from build123d import *
from OCP.BRepFilletAPI import BRepFilletAPI_MakeChamfer

# Parameters (mm, degrees)
SKETCH_1_W          = 24
SKETCH_1_H          = 107
EXTRUDE_1_DEPTH     = 15
EXTRUDE_2_DEPTH     = 9
SKETCH_3_W          = 20
SKETCH_3_H          = 20
EXTRUDE_4_DEPTH     = 40
SKETCH_4_W          = 24
SKETCH_4_H          = 12
EXTRUDE_6_DEPTH     = 25
CHAMFER_2_SIZE      = 2
SKETCH_5_W          = 16
SKETCH_5_H          = 16
SKETCH_5_R          = 3
EXTRUDE_7_DEPTH     = 10
CHAMFER_3_SIZE      = 2
SKETCH_6_W          = 24
SKETCH_6_H          = 12
SKETCH_6_R          = 2.1
EXTRUDE_8_DEPTH     = 12
EXTRUDE_START       = -12
SKETCH_7_W          = 24
SKETCH_7_H          = 12
SKETCH_7_R          = 2.1
EXTRUDE_9_DEPTH     = 12
FILLET_1_R          = 10
CHAMFER_4_SIZE      = 16
CHAMFER_4_SIZE2     = 27.712812921
CUT_EXTRUDE_1_DEPTH = 12
FILLET_2_R          = 2


with BuildPart() as part:
    # Эскиз1 → Бобышка-Вытянуть1 (new body)
    with BuildSketch(Plane(origin=(0, 0, 0), x_dir=(1, 0, 0), z_dir=(0, 1, 0))):
        with Locations((-12, 0)):
            Rectangle(SKETCH_1_W, SKETCH_1_H)
    extrude(amount=EXTRUDE_1_DEPTH)

    # Эскиз2 → Бобышка-Вытянуть2 (add)
    with BuildSketch(Plane(origin=(0, 15, 0), x_dir=(1, 0, 0), z_dir=(0, 1, 0))):
        Polygon((0, 0), (0, 41.5), (-24, 41.5), (-24, -41.5), (0, -41.5), align=None)
    extrude(amount=EXTRUDE_2_DEPTH)

    # Эскиз3 → Бобышка-Вытянуть4 (add)
    with BuildSketch(Plane(origin=(0, 0, 0), x_dir=(1, 0, 0), z_dir=(0, 1, 0))):
        Polygon((0, 53.5), (20, 41.5), (0, 41.5), align=None)
        with Locations((10, 31.5)):
            Rectangle(SKETCH_3_W, SKETCH_3_H)
        with Locations((10, -31.5)):
            Rectangle(SKETCH_3_W, SKETCH_3_H)
        Polygon((0, -41.5), (0, -53.5), (20, -41.5), align=None)
    extrude(amount=EXTRUDE_4_DEPTH)

    # Эскиз4 → Бобышка-Вытянуть6 (add)
    with BuildSketch(Plane(origin=(0, 15, 0), x_dir=(1, 0, 0), z_dir=(0, 1, 0))):
        with Locations((-12, 47.5)):
            Rectangle(SKETCH_4_W, SKETCH_4_H)
        with Locations((-12, -47.5)):
            Rectangle(SKETCH_4_W, SKETCH_4_H)
    extrude(amount=EXTRUDE_6_DEPTH)

    # Фаска2
    chamfer_2_edges = [part.edges().sort_by_distance(p)[0] for p in [
        (0, 12, -21.5),
        (20, 20, -21.5),
        (0, 12, 21.5),
        (20, 20, 21.5),
    ]]
    chamfer(chamfer_2_edges, length=CHAMFER_2_SIZE)

    # Эскиз5 → Бобышка-Вытянуть7 (add)
    # profile 1 of 3: a face of its own
    with BuildSketch(Plane(origin=(0, 0, 0), x_dir=(1, 0, 0), z_dir=(0, 1, 0))):
        with Locations((-32, 45.5)):
            Rectangle(SKETCH_5_W, SKETCH_5_H)
        with Locations(Location((-32, 45.5, 0), (0, 0, 270))):
            Circle(SKETCH_5_R, mode=Mode.SUBTRACT)
    # profile 2 of 3: a face of its own
    with BuildSketch(Plane(origin=(0, 0, 0), x_dir=(1, 0, 0), z_dir=(0, 1, 0))):
        with Locations((-32, -45.5)):
            Rectangle(SKETCH_5_W, SKETCH_5_H)
        with Locations(Location((-32, -45.5, 0), (0, 0, 270))):
            Circle(SKETCH_5_R, mode=Mode.SUBTRACT)
    # profile 3 of 3: a face of its own
    with BuildSketch(Plane(origin=(0, 0, 0), x_dir=(1, 0, 0), z_dir=(0, 1, 0))):
        with Locations((8, 0)):
            Rectangle(SKETCH_5_W, SKETCH_5_H)
        with Locations(Location((8, 0, 0), (0, 0, 270))):
            Circle(SKETCH_5_R, mode=Mode.SUBTRACT)
    extrude(amount=EXTRUDE_7_DEPTH)

    # Фаска3
    chamfer_3_edges = [part.edges().sort_by_distance(p)[0] for p in [
        (-24, 10, -45.5),
        (-24, 10, 45.5),
        (0, 10, 0),
    ]]
    chamfer(chamfer_3_edges, length=CHAMFER_3_SIZE)

    # Эскиз6 → Бобышка-Вытянуть8 (add)
    with BuildSketch(Plane(origin=(0, 0, -53.5), x_dir=(-1, 0, 0), z_dir=(0, 0, -1))):
        with Locations((12, 46)):
            Rectangle(SKETCH_6_W, SKETCH_6_H)
        with Locations((12, 46)):
            Circle(SKETCH_6_R, mode=Mode.SUBTRACT)
    extrude(amount=-EXTRUDE_8_DEPTH)

    # Эскиз7 → Бобышка-Вытянуть9 (add)
    with BuildSketch(Plane.XY.offset(53.5).offset(EXTRUDE_START)):
        with Locations((-12, 46)):
            Rectangle(SKETCH_7_W, SKETCH_7_H)
        with Locations(Location((-12, 46, 0), (0, 0, 180))):
            Circle(SKETCH_7_R, mode=Mode.SUBTRACT)
    extrude(amount=EXTRUDE_9_DEPTH)

    # Скругление1
    fillet_1_edges = [part.edges().sort_by_distance(p)[0] for p in [
        (0, 52, -47.5),
        (-24, 52, -47.5),
        (-24, 52, 47.5),
        (0, 52, 47.5),
    ]]
    fillet(fillet_1_edges, radius=FILLET_1_R)

    # Фаска4: one chamfer whose edges measure the first distance from different faces: ONE call of the kernel's chamfer builder (chamfer() names one face for all edges)
    chamfer_4_edges_1 = [part.edges().sort_by_distance(p)[0] for p in [
        (20, 40, 32.5),
    ]]
    chamfer_4_side_1 = [part.faces().sort_by_distance(p)[0] for p in [
        (9.191763192, 40, 34.779279279),
    ]]
    chamfer_4_edges_2 = [part.edges().sort_by_distance(p)[0] for p in [
        (20, 40, -32.5),
    ]]
    chamfer_4_side_2 = [part.faces().sort_by_distance(p)[0] for p in [
        (9.191763192, 40, -34.779279279),
    ]]
    chamfer_4 = BRepFilletAPI_MakeChamfer(part.part.solid().wrapped)
    for e in chamfer_4_edges_1:
        chamfer_4.Add(CHAMFER_4_SIZE, CHAMFER_4_SIZE2, e.wrapped, chamfer_4_side_1[0].wrapped)  # the first distance lies on this face
    for e in chamfer_4_edges_2:
        chamfer_4.Add(CHAMFER_4_SIZE, CHAMFER_4_SIZE2, e.wrapped, chamfer_4_side_2[0].wrapped)  # the first distance lies on this face
    add(Compound.cast(chamfer_4.Shape()), mode=Mode.REPLACE)

    # Эскиз8 → Вырез-Вытянуть1 (cut)
    with BuildSketch(Plane(origin=(0, 24, 0), x_dir=(1, 0, 0), z_dir=(0, 1, 0))):
        Polygon((-24, 0), (-24, 30), (-12, 20), (-12, 0), (-12, -20), (-24, -30), align=None)
    extrude(amount=-CUT_EXTRUDE_1_DEPTH, mode=Mode.SUBTRACT)

    # Скругление2
    fillet_2_edges = [part.edges().sort_by_distance(p)[0] for p in [
        (-24, 12, 0),
        (-12, 24, 0),
    ]]
    fillet(fillet_2_edges, radius=FILLET_2_R)


solid = part.part
Part model, mm, in its own coordinate system. A direction names the side the tool comes from. Give positions to 0.01 mm unless a question says otherwise; leave off trailing zeros. Order: outer loops, then holes, each group sorted by start corner. A loop starts at its lowest first (then second) coordinate and runs counter-clockwise, first axis right, second up. Notation, with made-up numbers: (86, 65) -> (109, 65) arc R25 ccw to (109, 96) -> close; hole circle Ø10 at (4.25, 73.25). An arc over 180 degrees is marked (long way). Use one line per item in the form item = value.
(1) Pull direction Z, two halves, no side cores. Call faces 1 (the face through (-32, 5, 37.5)), 2 (the face through (-16, 21, 53.5)), 3 (the face through (-21.15, 48.99, -47.42)): +Z half, -Z half, draft (parallel to the pull), parting line (faces both ways), or undercut.
Solution:
face_1 = undercut
face_2 = +Z half
face_3 = draft
(2) Flat gauge pins, fed straight in: P1, Ø4, axis at x = -17, z = 16, coming from the -Y side; P2, Ø4.5, axis at x = 2.5, z = -42, coming from the +Y side; P3, Ø0.6, axis at y = 41, z = 48.5, coming from the +X side; P4, Ø13, axis at x = -11.5, z = -3, coming from the +Y side. Where does each tip first touch, or does it go through?
Solution:
P1 = 0
P2 = 40
P3 = 0
P4 = 24
(3) Saw through at A-A (z = 46). Write the cut outline in (x, y).
Solution:
outline = (-40, 0) -> (-34.96, 0) -> (-34.96, 10) -> (-40, 10) -> close; (-29.04, 0) -> (12.5, 0) -> (12.5, 25.28) -> (4, 40) -> (0, 40) -> (0, 42) arc R10 ccw to (-10, 52) -> (-14, 52) arc R10 ccw to (-24, 42) -> (-24, 12) -> (-26, 10) -> (-29.04, 10) -> close; hole circle Ø4.2 at (-12, 46)
(4) Tool access for faces 4 (the face through (-35, 10, -44)), 5 (the face through (12, 10, 0)), 6 (the face through (-11.4, 23.43, -0.28)), 7 (the face through (19, 7.8, -22.5)), 8 (the face through (-10, 0, -1)): list every direction of +Z, -Z, +X, -X, +Y, -Y with a clear straight run to the whole face (end or side of a thin tool).
Solution:
face_4 = +Z, -Z, -X, +Y
face_5 = +X, +Y
face_6 = -X, +Y
face_7 = +X, +Y, -Y
face_8 = +Z, -Z, +X, -X, -Y
(5) Saw through at D-D (z = 0). Write the cut outline in (x, y).
Solution:
outline = (-24, 0) -> (5, 0) -> (5, 10) -> (2, 10) -> (0, 12) -> (0, 24) -> (-10, 24) arc R2 ccw to (-12, 22) -> (-12, 12) -> (-22, 12) arc R2 ccw to (-24, 10) -> close; (11, 0) -> (16, 0) -> (16, 10) -> (11, 10) -> close
(6) Saw through at B-B (x = -32). Write the cut outline in (y, z).
Solution:
outline = (0, -53.5) -> (10, -53.5) -> (10, -48.5) -> (0, -48.5) -> close; (0, -42.5) -> (10, -42.5) -> (10, -37.5) -> (0, -37.5) -> close; (0, 37.5) -> (10, 37.5) -> (10, 42.5) -> (0, 42.5) -> close; (0, 48.5) -> (10, 48.5) -> (10, 53.5) -> (0, 53.5) -> close
(7) Saw through at C-C (y = 5.5). Write the cut outline in (x, z), then the cut area to 3 significant figures.
Solution:
outline = (-40, -53.5) -> (0, -53.5) -> (20, -41.5) -> (20, -23.5) -> (18, -21.5) -> (2, -21.5) -> (0, -19.5) -> (0, -8) -> (16, -8) -> (16, 8) -> (0, 8) -> (0, 19.5) -> (2, 21.5) -> (18, 21.5) -> (20, 23.5) -> (20, 41.5) -> (0, 53.5) -> (-40, 53.5) -> (-40, 37.5) -> (-24, 37.5) -> (-24, -37.5) -> (-40, -37.5) -> close; hole circle Ø6 at (-32, -45.5); hole circle Ø6 at (-32, 45.5); hole circle Ø6 at (8, 0)
area = 4,290 mm²
(8) Drill centre lines: line 1 (Z direction, x = -16, y = 49.5); line 2 (Y direction, x = -12.5, z = 5); line 3 (Y direction, x = -12, z = -43.75). Where is each one in solid material? Low to high. Write a range as from..to.
Solution:
line_1 = -53.5..-41.5, 41.5..53.5
line_2 = 0..12
line_3 = 0..43.9, 48.1..52
